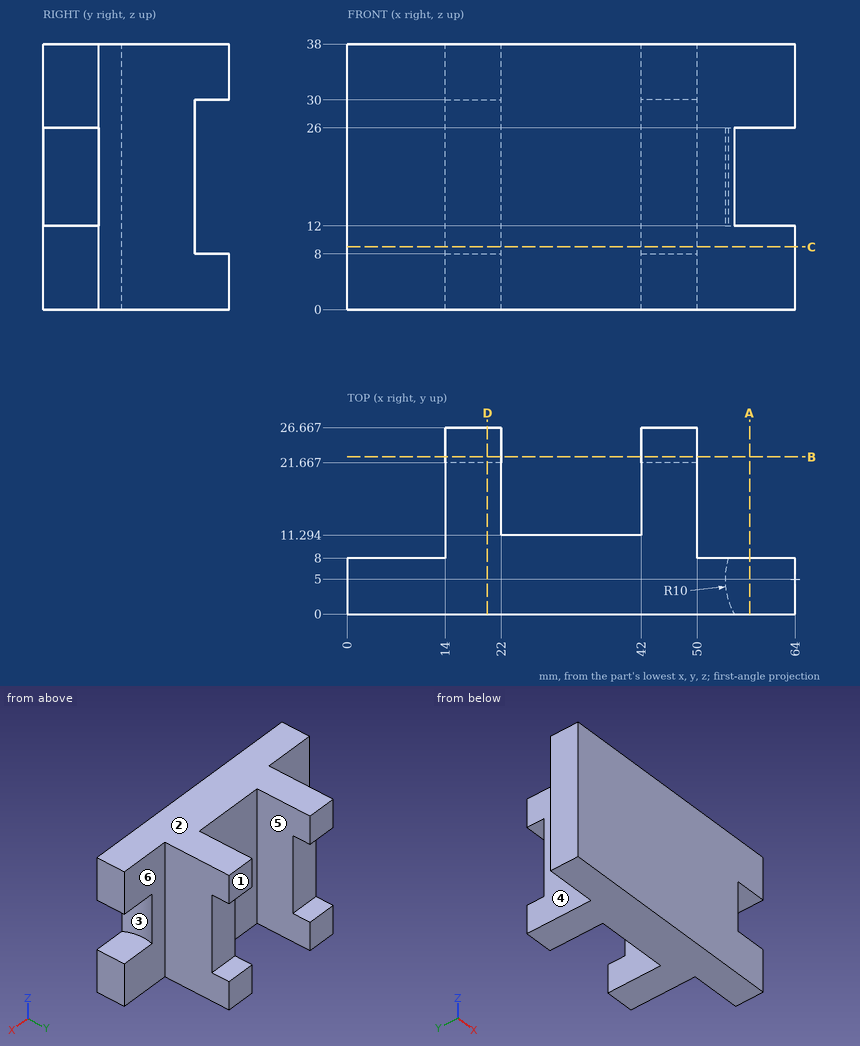
Input: dimensioned drawing with shaded views. Units: mm. Origin: part minimum x, y, z. A direction names the side the tool comes from. Coordinates: 2 decimals unless noted, no trailing zeros. Loops run counter-clockwise (first coordinate to the right, second up) from the corner with the lowest first, then second, coordinate; pieces in that order, holes last. Notation, with made-up numbers: M -14,85.5 L 17,85.5 A16 ccw 17,93.5 Z; hole C 54.25,39.25 d11. An arc over 180 degrees is marked long. Use a Markdown table: item, result. Add a question column.
1) Set-up query: the marked faces 4, 5 and 6. Return all of +Z, -Z, +X, -X, +Y, -Y with unobstructed straight access to the full face (end or side cutting, diameter ignored); none if empty.
2) Section D-D, the plane x = 20. Return the cut outline in (y, z).
3) Line query: L1, parallel to X at y = 20.5, z = 33; L2, parallel to Z at x = 42.5, y = 25.25; L3, parallel to Y at x = 37.5, z = 31. Output: solid intervals per line, ascending. Write a range as from..to.
4) Section A-A, the plane x = 57.5. Return the cut outline in (y, z), plus the area to 3 significant figures.
5) Draft query along Y for the marked faces 1, 2 and 3. Return one class per face: +Y half, -Y half, draft (parallel to the pull), parting line (faces both ways), or undercut.
6) Section B-B, the plane y = 22.5. Return the cut outline in (x, z).
7) Pin query (flat end, axial travel): P1, Ø12.5, axis at y = 18.5, z = 14.5, coming from the +X side; P2, Ø4.5, axis at y = 16, z = 14, coming from the -X side; P3, Ø11, axis at x = 60.5, z = 18, coming from the +Y side. Return the tip coordinate at first contact, or that it passes through.
8) Section C-C, the plane z = 9. Return the cut outline in (x, y).
Answer below:
| question | item | result |
|---|---|---|
| 1 | face 4 | +Z, -Z, -X, +Y |
| 1 | face 5 | +Z, -Z, +Y |
| 1 | face 6 | +Z, -Z, +X, +Y |
| 2 | outline | M 0,0 L 26.67,0 L 26.67,8 L 21.67,8 L 21.67,30 L 26.67,30 L 26.67,38 L 0,38 Z |
| 3 | L1 | 14..22, 42..50 |
| 3 | L2 | 0..8, 30..38 |
| 3 | L3 | 0..11.29 |
| 4 | outline | M 0,0 L 8,0 L 8,12 L 0,12 Z; M 0,26 L 8,26 L 8,38 L 0,38 Z |
| 4 | area | 192 mm2 |
| 5 | face 1 | +Y half |
| 5 | face 2 | draft |
| 5 | face 3 | undercut |
| 6 | outline | M 14,0 L 22,0 L 22,8 L 14,8 Z; M 14,30 L 22,30 L 22,38 L 14,38 Z; M 42,0 L 50,0 L 50,8 L 42,8 Z; M 42,30 L 50,30 L 50,38 L 42,38 Z |
| 7 | P1 | x = 50 |
| 7 | P2 | x = 14 |
| 7 | P3 | y = 0.64 |
| 8 | outline | M 0,0 L 64,0 L 64,8 L 50,8 L 50,21.67 L 42,21.67 L 42,11.29 L 22,11.29 L 22,21.67 L 14,21.67 L 14,8 L 0,8 Z |
